The model under review builds one solid part; all positions refer to its coordinate system, in mm. Face numbers are marked on the shaded views. A direction names the side the tool comes from. Give positions to 0.01 mm unless a question says otherwise; leave off trailing zeros. Loops run counter-clockwise (first coordinate to the right, second up) from the corner with the lowest first, then second, coordinate; pieces in that order, holes last. Notation, with made-up numbers: (51, 44) - (96, 44) arc R17 cw to (96, 67) - close; hole circle Ø8 at (89.25, 25). An arc over 180 degrees is marked (long way). Return JSON: item names as keys, results as strings. Group by question number.
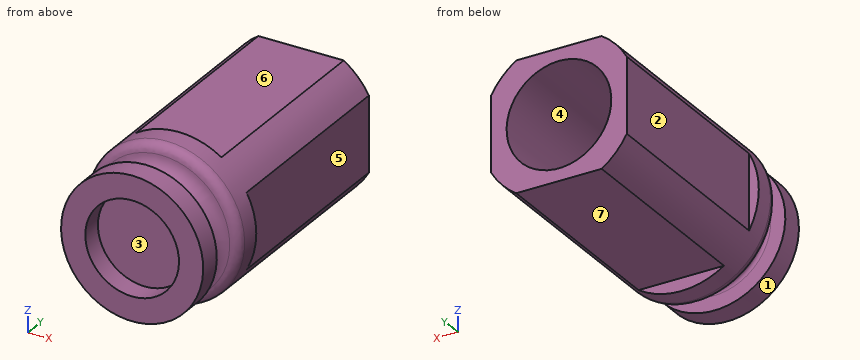
```python
from build123d import *

# Parameters (mm, degrees)
SKETCH_1_R                 = 22
EXTRUDE_1_DEPTH            = 15
SKETCH_2_R                 = 14.5
CUT_EXTRUDE_2_DEPTH        = 6.5
SKETCH_4_R                 = 25
SKETCH_4_R_2               = 16.5
CUT_EXTRUDE_1_DEPTH        = 8
SKETCH_5_R                 = 24
SKETCH_5_R_2               = 16.2
EXTRUDE_4_DEPTH            = 72
FILLET_1_R                 = 1
FILLET_2_R                 = 5
FILLET_3_R                 = 3
CUT_EXTRUDE_2_2_DEPTH      = 50
CUT_EXTRUDE_2_2_DEPTH_BACK = 26
CUT_EXTRUDE_2_2_START      = 50
SKETCH_6_W                 = 42
SKETCH_6_H                 = 40.064513034


with BuildPart() as part:
    # Эскиз1 → Вытянуть1 (new body)
    with BuildSketch(Plane(origin=(0, 0, 0), x_dir=(1, 0, 0), z_dir=(0, 1, 0))):
        with Locations(Location((0, 0, 0), (0, 0, 270))):
            Circle(SKETCH_1_R)
    extrude(amount=EXTRUDE_1_DEPTH)

    # Эскиз2 → Cut-Extrude 2 (cut)
    with BuildSketch(Plane.XZ):
        with Locations(Location((0, 0, 0), (0, 0, 270))):
            Circle(SKETCH_2_R)
    extrude(amount=-CUT_EXTRUDE_2_DEPTH, mode=Mode.SUBTRACT)

    # Эскиз4 → Вырез-Вытянуть1 (cut)
    with BuildSketch(Plane(origin=(0, 15, 0), x_dir=(1, 0, 0), z_dir=(0, 1, 0))):
        Circle(SKETCH_4_R)
        with Locations(Location((0, 0, 0), (0, 0, 270))):
            Circle(SKETCH_4_R_2, mode=Mode.SUBTRACT)
    extrude(amount=-CUT_EXTRUDE_1_DEPTH, mode=Mode.SUBTRACT)

    # Эскиз5 → Вытянуть4 (add)
    with BuildSketch(Plane(origin=(0, 15, 0), x_dir=(1, 0, 0), z_dir=(0, 1, 0))):
        with Locations(Location((0, 0, 0), (0, 0, 270))):
            Circle(SKETCH_5_R)
        with Locations(Location((0, 0, 0), (0, 0, 270))):
            Circle(SKETCH_5_R_2, mode=Mode.SUBTRACT)
    extrude(amount=EXTRUDE_4_DEPTH)

    # Скругление1
    fillet_1_edges = [part.edges().sort_by_distance(p)[0] for p in [
        (0, 7, -16.5),
    ]]
    fillet(fillet_1_edges, radius=FILLET_1_R)

    # Скругление2
    fillet_2_edges = [part.edges().sort_by_distance(p)[0] for p in [
        (0, 15, -16.5),
    ]]
    fillet(fillet_2_edges, radius=FILLET_2_R)

    # Скругление3
    fillet_3_edges = [part.edges().sort_by_distance(p)[0] for p in [
        (0, 15, -24),
    ]]
    fillet(fillet_3_edges, radius=FILLET_3_R)

    # Эскиз6 → Cut-Extrude 2 2 (cut, two sides: drawn at the far end of the back side and taken through both)
    with BuildSketch(Plane(origin=(0, 0, 0), x_dir=(1, 0, 0), z_dir=(0, 1, 0)).offset(CUT_EXTRUDE_2_2_START - CUT_EXTRUDE_2_2_DEPTH_BACK)):
        Polygon((21, 29.701884449), (36.425926694, 29.701884449), (36.425926694, -29.522725679), (-36.425926694, -29.522725679), (-36.425926694, 29.701884449), (-21, 29.701884449), align=None)
        Rectangle(SKETCH_6_W, SKETCH_6_H, mode=Mode.SUBTRACT)
    extrude(amount=CUT_EXTRUDE_2_2_DEPTH + CUT_EXTRUDE_2_2_DEPTH_BACK, mode=Mode.SUBTRACT)


solid = part.part
```
1) We need section A-A, the plane y = 71. Write out the cut boundary in (x, z).
2) For pin 1 Ø1.5 at (x, z) = (-22, 4.5) entering from +Y; pin 2 Ø7 at (y, z) = (67.5, -3) entering from +X; pin 3 Ø3.5 at (x, z) = (22.5, 3.5) entering from +Y; pin 4 Ø10 at (x, z) = (-3.5, -4.5) entering from +Y, all flat-tipped, find the tip position at first contact; note any pin that passes through.
3) Tool access review of the marked faces 4, 5, 6 and 7: name each direction out of +Z, -Z, +X, -X, +Y, -Y from which nothing blocks a thin tool from reaching the whole face with its end or side.
4) To check wall thickness, follow line 1 (X direction, y = 4, z = 0); line 2 (Y direction, x = 5, z = 5); line 3 (Y direction, x = 4.5, z = -20.5). State the ranges of each line that lie inside material, in increasing order.
5) Draft analysis for pull direction Z (two halves, no side actions). For the marked faces 1, 2 and 3, state which applies: +Z half, -Z half, draft (parallel to the pull), parting line (faces both ways), or undercut.
Findings:
{
 "1": {"outline": "(-21, -11.62) arc R24 ccw to (-13.22, -20.03) - (13.22, -20.03) arc R24 ccw to (21, -11.62) - (21, 11.62) arc R24 ccw to (13.22, 20.03) - (-13.22, 20.03) arc R24 ccw to (-21, 11.62) - close; hole circle Ø32.4 at (0, 0)"},
 "2": {"pin 1": "stops at y = 24", "pin 2": "stops at x = 21", "pin 3": "stops at y = 87", "pin 4": "stops at y = 15"},
 "3": {"face 4": "+Y", "face 5": "+Z, -Z, +X, +Y", "face 6": "+Z, +X, -X, +Y", "face 7": "-Z, +X, -X, +Y"},
 "4": {"line 1": "x = -22 to -14.5, 14.5 to 22", "line 2": "y = 6.5 to 15", "line 3": "y = 0 to 7, 14.97 to 24"},
 "5": {"face 1": "parting line", "face 2": "draft", "face 3": "undercut"}
}
